Job drawing, mm, ordinate dimensions from the low corner. One solid piece. A direction names the side the tool comes from. Give positions to 0.01 mm unless a question says otherwise; leave off trailing zeros. Loops run counter-clockwise (first coordinate to the right, second up) from the corner with the lowest first, then second, coordinate; pieces in that order, holes last.
Item 1: Saw through at C-C on z = 55.5. Give the cut face in (x, y) (3 decimals), plus the area to 3 significant figures.
Item 2: Probe probe 1 along Y at (x, z) = (8.25, 57.5); probe 2 along Y at (x, z) = (8, 3.9); probe 3 along X at (y, z) = (5.5, 9.5). List the from-to ranges inside material, lowest first.
Item 3: Mould opens along X. For the marked faces 3, 4, 5 and 6 say: released by +X, released by -X, zero draft, split by the parting line, or undercut.
Item 4: Which spindle directions (+Z, -Z, +X, -X, +Y, -Y) get a long thin tool onto all of the face, cutting with end or side? Do the marked faces 1 and 2. Say none if no direction does.
Item 5: Saw through at A-A on y = 8. Give the cut face in (x, z) (3 decimals), plus the area to 3 significant figures.
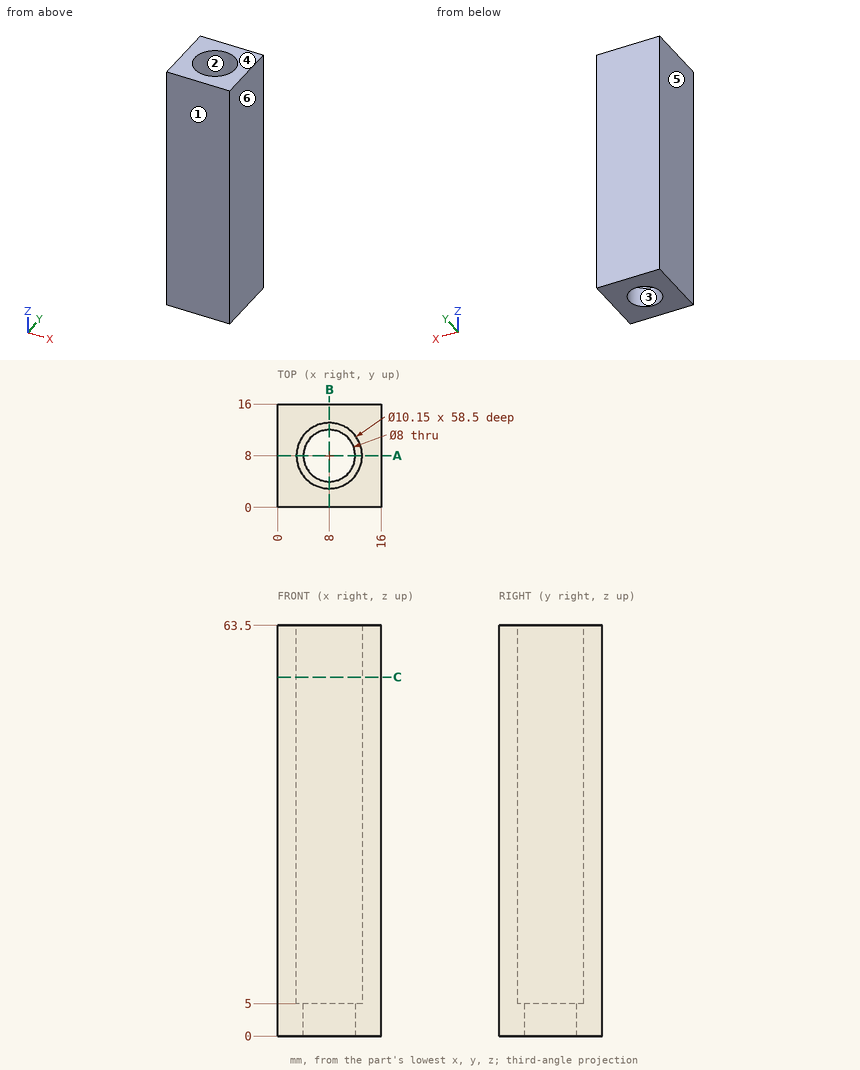
Results below:
1. outline: (0, 0) - (16, 0) - (16, 16) - (0, 16) - close; hole circle Ø10.15 at (8, 8)
1. area: 175 mm2
2. probe 1: y = 0 to 2.93, 13.07 to 16
2. probe 2: y = 0 to 4, 12 to 16
2. probe 3: x = 0 to 3.58, 12.42 to 16
3. face 3: undercut
3. face 4: zero draft
3. face 5: released by -X
3. face 6: released by +X
4. face 1: +Z, -Z, +X, -X, -Y
4. face 2: +Z
5. outline: (0, 0) - (4, 0) - (4, 5) - (2.925, 5) - (2.925, 63.5) - (0, 63.5) - close; (12, 0) - (16, 0) - (16, 63.5) - (13.075, 63.5) - (13.075, 5) - (12, 5) - close
5. area: 382 mm2
